Print and shaded views of the part. All mm, measured from the part's lowest x, y and z. A direction names the side the tool comes from. Round coordinates to 2 decimals unless told otherwise and drop trailing zeros. Loops run counter-clockwise (first coordinate to the right, second up) from the corner with the lowest first, then second, coordinate; pieces in that order, holes last. Notation, with made-up numbers: (-31.75, 48.5) - (18.25, 48.5) arc R8 cw to (18.25, 61.5) - close; hole circle Ø1 at (-20.75, 89). An arc over 180 degrees is marked (long way). Use one line per item in the form item = value.
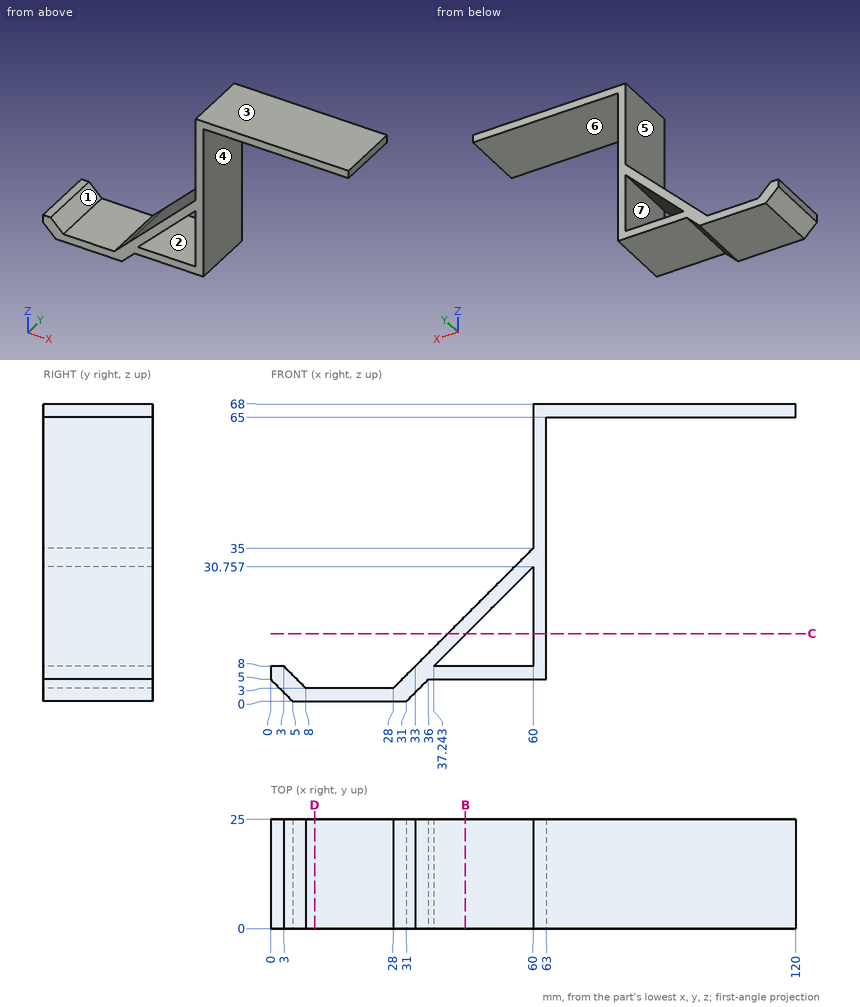
1. Flat gauge pins, fed straight in: pin 1 (3 mm diameter, centred on x = 57.5, y = 7.5, fed in from +Z); pin 2 (2.5 mm diameter, centred on x = 1, y = 14, fed in from +Z); pin 3 (7.5 mm diameter, centred on x = 98.5, y = 8.5, fed in from -Z); pin 4 (12 mm diameter, centred on x = 33.5, z = 23.5, fed in from -Y). Where does each tip first touch, or does it go through?
Geometry check:
pin_1 = 34
pin_2 = 8
pin_3 = 65
pin_4 = through
2. Cut at C-C, the plane z = 15.5. Give the cut face in (x, y).
Geometry check:
outline = (40.5, 0) - (44.74, 0) - (44.74, 25) - (40.5, 25) - close; (60, 0) - (63, 0) - (63, 25) - (60, 25) - close
3. Cut at B-B, the plane x = 44.5. Give the cut face in (y, z).
Geometry check:
outline = (0, 5) - (25, 5) - (25, 8) - (0, 8) - close; (0, 15.26) - (25, 15.26) - (25, 19.5) - (0, 19.5) - close
4. Tool access for the marked faces 1, 2, 3 and 4: list every direction of +Z, -Z, +X, -X, +Y, -Y with a clear straight run to the whole face (end or side of a thin tool).
Geometry check:
face_1 = +Z, +Y, -Y
face_2 = +Y, -Y
face_3 = +Z, +X, -X, +Y, -Y
face_4 = -Z, +X, +Y, -Y
5. Wall check: probe 1 along X at (y, z) = (20.5, 6); probe 2 along X at (y, z) = (15.25, 47); probe 3 along Z at (x, y) = (71, 5). Give the ranges that are in metal, low to high.
Geometry check:
probe_1 = 0 to 5, 31 to 63
probe_2 = 60 to 63
probe_3 = 65 to 68
6. Cut at D-D, the plane x = 10. Give the cut face in (y, z), plus the area to 3 significant figures.
Geometry check:
outline = (0, 0) - (25, 0) - (25, 3) - (0, 3) - close
area = 75.0 mm^2
7. Pull direction X, two halves, no side cores. Call the marked faces 5, 6 and 7: +X half, -X half, draft (parallel to the pull), parting line (faces both ways), or undercut.
Geometry check:
face_5 = -X half
face_6 = draft
face_7 = undercut
